Study the drawing (mm; zero at the part's minimum x, y, z) and answer. Coordinates: 2 decimals unless noted, no trailing zeros.
1. Flat-ended cylindrical pins translate along their axes: pin 1 Ø4 at (x, z) = (153, 280) entering from -Y; pin 2 Ø3 at (x, y) = (38, 4.5) entering from +Z. Find the tip coordinate at first contact, or state that the pin passes through.
2. Find the intervals of material crossed by probe 1 along Z at (x, y) = (8.5, 2.6); probe 2 along X at (y, z) = (3.25, 280); probe 3 along X at (y, z) = (1.45, 278), in increasing order.
3. The part is cut by section A-A, the plane y = 3.1. Count the separate pieces of the cut face and the enclosed holes in it, then the cut area to 3 significant figures.
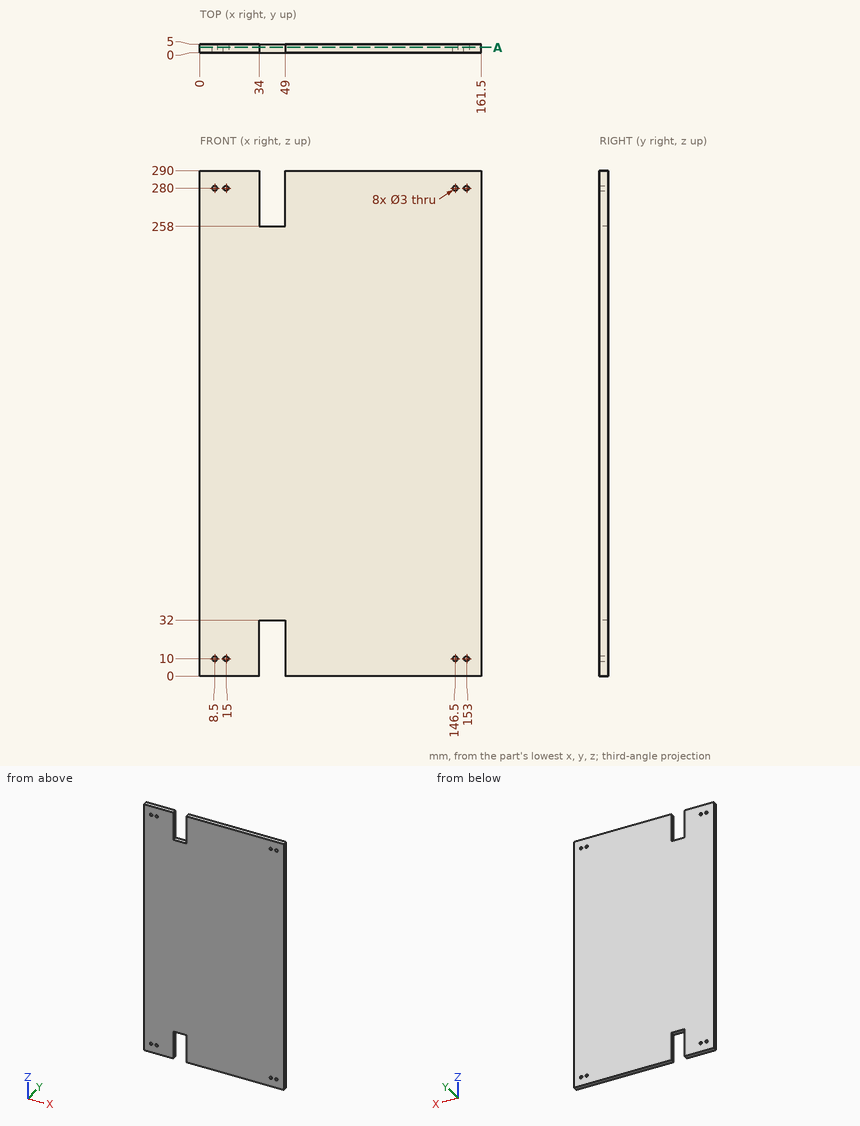
Geometry says:
1. pin 1: stops at y = 0
1. pin 2: stops at z = 258
2. probe 1: z = 0 to 8.5, 11.5 to 278.5, 281.5 to 290
2. probe 2: x = 0 to 7, 10 to 13.5, 16.5 to 34, 49 to 145, 148 to 151.5, 154.5 to 161.5
2. probe 3: x = 0 to 34, 49 to 161.5
3. separate pieces: 1
3. enclosed holes: 8
3. area: 45,800 mm2
